Read the model definition and answer for the solid it produces. Units are mm, in the model's axes. A direction names the side the tool comes from. Coordinates: 2 decimals unless noted, no trailing zeros. Write each loop counter-clockwise with the first axis right and the second up, starting at its lowest first coordinate (ties: lowest second). Pieces come first, ordered by that corner, then holes. Notation, with made-up numbers: (-29.5, 1) -> (-17.5, 1) arc R16 ccw to (-17.5, 31) -> close; hole circle Ø5 at (64.5, 36.25). An arc over 180 degrees is marked (long way). Write item = value, one per line. Start each with the question number.
1) Section A-A (y = 21.5) is taken. Determine the outline of the cut face in (x, z), plus the area to 3 significant figures.
2) A flat-ended cylindrical pin translates along its axis: pin 1 Ø2 at (x, y) = (214.5, 36.5) entering from -Z. Find the tip coordinate at first contact, or state that the pin passes through.
3) A tool of negligible diameter and unlimited length cuts with its end or side. For faces 4 (the face through (264, 25, 2)), 5 (the face through (130, -3, -151)), 6 (the face through (10, 24, 2)), from which of +Z, -Z, +X, -X, +Y, -Y can it reach the whole face along a straight path? Write none if from no direction.
4) For a pull along Z with two mould halves and no side action, classify faces 1 (the face through (134, 0, -2)), 2 (the face through (134, 8, -166)), 3 (the face through (133.853, -8.754, -158.395)) as released by +Z, released by -Z, zero draft, split by the parting line, or undercut.
5) Section B-B (x = 147) is taken. Determine the outline of the cut face in (y, z), plus the area to 3 significant figures.
6) Section C-C (z = 15) is taken. Determine the outline of the cut face in (x, y).
7) Section D-D (x = 119) is taken. Determine the outline of the cut face in (y, z), plus the area to 3 significant figures.
8) Find the intervals of material crossed by line 1 along Y through (x, z) = (214, -31.5); line 2 along X through (y, z) = (34, -14.5); line 3 along Z through (x, y) = (208, -2.5), in increasing order. Write a range as from..to.
from build123d import *

# Parameters (mm, degrees)
SKETCH1_W           = 244
SKETCH1_H           = 29
BOSS_EXTRUDE1_DEPTH = 166
SKETCH3_W           = 264
SKETCH3_H           = 30.556086773
CUT_EXTRUDE2_DEPTH  = 151
SKETCH4_W           = 264
SKETCH4_H           = 302
BOSS_EXTRUDE2_DEPTH = 10


with BuildPart() as part:
    # Sketch1 → Boss-Extrude1 (new, symmetric)
    with BuildSketch(Plane.XY):
        with BuildLine():
            Line((0, 0), (0, 49))
            Line((0, 49), (264, 49))
            Line((264, 49), (264, 0))
            ThreePointArc((264, 0), (132, -8.755804433), (0, 0))
        make_face()
        with Locations((132, 24.5)):
            Rectangle(SKETCH1_W, SKETCH1_H, mode=Mode.SUBTRACT)
    extrude(amount=BOSS_EXTRUDE1_DEPTH, both=True)

    # Sketch3 → Cut-Extrude2 (cut, symmetric)
    with BuildSketch(Plane.XY):
        with Locations((132, -5.278043387)):
            Rectangle(SKETCH3_W, SKETCH3_H)
    extrude(amount=CUT_EXTRUDE2_DEPTH, both=True, mode=Mode.SUBTRACT)

    # Sketch4 → Boss-Extrude2 (add)
    with BuildSketch(Plane(origin=(0, 10, 0), x_dir=(-1, 0, 0), z_dir=(0, -1, 0))):
        with Locations((-132, 0)):
            Rectangle(SKETCH4_W, SKETCH4_H)
    extrude(amount=BOSS_EXTRUDE2_DEPTH)


solid = part.part
Answer key:
q1.outline = (0, -166) -> (10, -166) -> (10, 166) -> (0, 166) -> close; (254, -166) -> (264, -166) -> (264, 166) -> (254, 166) -> close
q1.area = 6,640 mm^2
q2.pin_1 = through
q3.face_4 = +Z, -Z, +X, +Y, -Y
q3.face_5 = +X, -X, -Y
q3.face_6 = +Z, -Z
q4.face_1 = undercut
q4.face_2 = released by -Z
q4.face_3 = zero draft
q5.outline = (-8.64, -166) -> (10, -166) -> (10, 166) -> (-8.64, 166) -> (-8.64, 151) -> (0, 151) -> (0, -151) -> (-8.64, -151) -> close; (39, -166) -> (49, -166) -> (49, 166) -> (39, 166) -> close
q5.area = 6,900 mm^2
q6.outline = (0, 0) -> (264, 0) -> (264, 49) -> (0, 49) -> close; hole (10, 10) -> (254, 10) -> (254, 39) -> (10, 39) -> close
q7.outline = (-8.67, -166) -> (10, -166) -> (10, 166) -> (-8.67, 166) -> (-8.67, 151) -> (0, 151) -> (0, -151) -> (-8.67, -151) -> close; (39, -166) -> (49, -166) -> (49, 166) -> (39, 166) -> close
q7.area = 6,900 mm^2
q8.line_1 = 0..10, 39..49
q8.line_2 = 0..10, 254..264
q8.line_3 = -166..-151, 151..166
